Design review of the part built by this model. Coordinates are the model's own, in mm. A direction names the side the tool comes from. Round coordinates to 2 decimals unless told otherwise and drop trailing zeros. Write each loop counter-clockwise with the first axis right and the second up, starting at its lowest first coordinate (ties: lowest second). Pieces come first, ordered by that corner, then holes. Notation, with made-up numbers: M 0.5,17.25 L 5.5,17.25 A22 ccw 5.5,28.25 Z; hole C 85,-23.5 d3. An arc over 180 degrees is marked long. One line per question, with ' | ' between items. Start each with the question number.
Item 1: Add section D-D, the plane x = -26.5. State the section outline as (y, z) points, and give its area (4 significant figures).
Item 2: Add section A-A, the plane x = 30. State the section outline as (y, z) points.
Item 3: Draft analysis for pull direction Y (two halves, no side actions). For faces 5 (the face through (2.48, -133.38, 63.01)), 6 (the face through (-5, -125, 15)), 7 (the face through (1, -135, 60)), 8 (the face through (29.779, -133.314, 10.93)), state which applies: released by +Y, released by -Y, zero draft, split by the parting line, or undercut.
Item 4: Insertion check: pin 1 Ø1.2 at (y, z) = (-134.5, 4.5) entering from +X; pin 2 Ø9.5 at (x, y) = (21, -137.5) entering from +Z; pin 3 Ø3.5 at (y, z) = (-134.5, 63.5) entering from +X. Each pin has a flat end and moves straight along its axis. Give the tip position at first contact, or say it passes through.
Item 5: For L1, parallel to X at y = -135, z = 10; L2, parallel to X at y = -142, z = 64; L3, parallel to Z at x = 18, y = -142.5, list the stretches that pass through material, from the lowest coordinate up.
Item 6: Add section B-B, the plane z = 62.5. State the section outline as (x, y) points, and give its area (3 significant figures).
Item 7: Add section C-C, the plane y = -130.5. State the section outline as (x, z) points, and give its area (3 significant figures).
Item 8: Machinability: for faces 1 (the face through (25, -134, 6)), 2 (the face through (-4, -134.9, 64.5)), 3 (the face through (-25, -134, 6)), 4 (the face through (4, -134.9, 64.5)), which of the approach directions +Z, -Z, +X, -X, +Y, -Y give a long, thin tool a straight path to every point of the face, cutting with its end or side? Answer none if there is none.
```python
from build123d import *

# Parameters (mm, degrees)
SKETCH_R        = 19.7
PAD011_DEPTH    = 20
SKETCH020_W     = 2
SKETCH020_H     = 18
POCKET001_DEPTH = 30
SKETCH021_R     = 1.7
HOLE001_DEPTH   = 25
SKETCH022_R     = 1.7
HOLE002_DEPTH   = 25
CHAMFER003_SIZE = 1


with BuildPart() as part:
    # Sketch → Pad011 (new body)
    with BuildSketch(Plane.XZ.offset(100)):
        with BuildLine():
            Line((-34.918445, 6), (-34.918445, 16))
            Line((-34.918445, 16), (-14.918445, 16))
            ThreePointArc((-4, 58.464319), (-23.243956, 40.776496), (-14.918445, 16))
            Line((-4, 58.464319), (-4, 66.464319))
            Line((-4, 66.464319), (4, 66.464319))
            Line((4, 58.464319), (4, 66.464319))
            ThreePointArc((14.918445, 16), (23.243956, 40.776496), (4, 58.464319))
            Line((34.918445, 16), (14.918445, 16))
            Line((34.918445, 6), (34.918445, 16))
            Line((15.75, 6), (34.918445, 6))
            Line((15.75, 2), (15.75, 6))
            Line((-15.75, 2), (15.75, 2))
            Line((-15.75, 6), (-15.75, 2))
            Line((-15.75, 6), (-34.918445, 6))
        make_face()
        with Locations((0, 34.8)):
            Circle(SKETCH_R, mode=Mode.SUBTRACT)
    extrude(amount=PAD011_DEPTH)

    # Sketch020 → Pocket001 (cut)
    with BuildSketch(Plane.XZ.offset(98)):
        with Locations((0, 59.399123)):
            Rectangle(SKETCH020_W, SKETCH020_H)
    extrude(amount=POCKET001_DEPTH, mode=Mode.SUBTRACT)

    # Sketch021 → Hole001 (cut)
    with BuildSketch(Plane.XY):
        with Locations((-30, -110)):
            Circle(SKETCH021_R)
        with Locations((30, -110)):
            Circle(SKETCH021_R)
    extrude(amount=HOLE001_DEPTH, mode=Mode.SUBTRACT)

    # Sketch022 → Hole002 (cut)
    with BuildSketch(Plane.YZ.offset(-10)):
        with Locations((-110, 62.5)):
            Circle(SKETCH022_R)
    extrude(amount=HOLE002_DEPTH, mode=Mode.SUBTRACT)

    # Chamfer003
    chamfer003_edges = [part.edges().sort_by_distance(p)[0] for p in [
        (-13.571846, -120, 20.520819),
        (14.279181, -120, 48.371846),
        (-4, -110, 58.464319),
        (4, -110, 58.464319),
        (34.918445, -110, 16),
        (-34.918445, -110, 16),
        (-34.918445, -120, 11),
        (34.918445, -120, 11),
        (-25.334222, -120, 6),
        (15.75, -120, 4),
        (25.334222, -120, 6),
    ]]
    chamfer(chamfer003_edges, length=CHAMFER003_SIZE)


with BuildPart() as part_1:
    # Body placement: moved
    add(part.part.moved(Location((0, -25, 0))))


solid = part_1.part
```
Computed values:
1) outline: M -145,7 L -144,6 L -125,6 L -125,16 L -145,16 Z | area: 199.5 mm^2
2) outline: M -145,7 L -144,6 L -136.7,6 L -136.7,16 L -145,16 Z; M -133.3,6 L -125,6 L -125,16 L -133.3,16 Z
3) face 5: undercut | face 6: released by +Y | face 7: zero draft | face 8: undercut
4) pin 1: stops at x = 15.75 | pin 2: stops at z = 52.46 | pin 3: stops at x = 4
5) L1: x = -34.92 to -31.7, -28.3 to 28.3, 31.7 to 34.92 | L2: x = -4 to -1, 1 to 4 | L3: z = 6 to 16, 18.93 to 26.79, 42.81 to 50.67
6) outline: M -4,-145 L -1,-145 L -1,-136.7 L -4,-136.7 Z; M -4,-133.3 L -1,-133.3 L -1,-125 L -4,-125 Z; M 1,-145 L 4,-145 L 4,-136.7 L 1,-136.7 Z; M 1,-133.3 L 4,-133.3 L 4,-125 L 1,-125 Z | area: 99.6 mm^2
7) outline: M -34.92,6 L -15.75,6 L -15.75,2 L 15.75,2 L 15.75,6 L 34.92,6 L 34.92,15 L 33.92,16 L 14.92,16 A24 ccw 4.98,58.28 L 4,59.46 L 4,66.46 L 1,66.46 L 1,54.47 A19.7 cw long -1,54.47 L -1,66.46 L -4,66.46 L -4,59.46 L -4.98,58.28 A24 ccw -14.92,16 L -33.92,16 L -34.92,15 Z | area: 1,350 mm^2
8) face 1: -Z, +X, +Y, -Y | face 2: +Z, -X, +Y, -Y | face 3: -Z, -X, +Y, -Y | face 4: +Z, +X, +Y, -Y
